Geometry: see drawing. Coordinates: mm, zero at the bounding-box minimum. A direction names the side the tool comes from. Coordinates: 2 decimals unless noted, no trailing zeros. Loops run counter-clockwise (first coordinate to the right, second up) from the corner with the lowest first, then second, coordinate; pieces in that order, holes last.
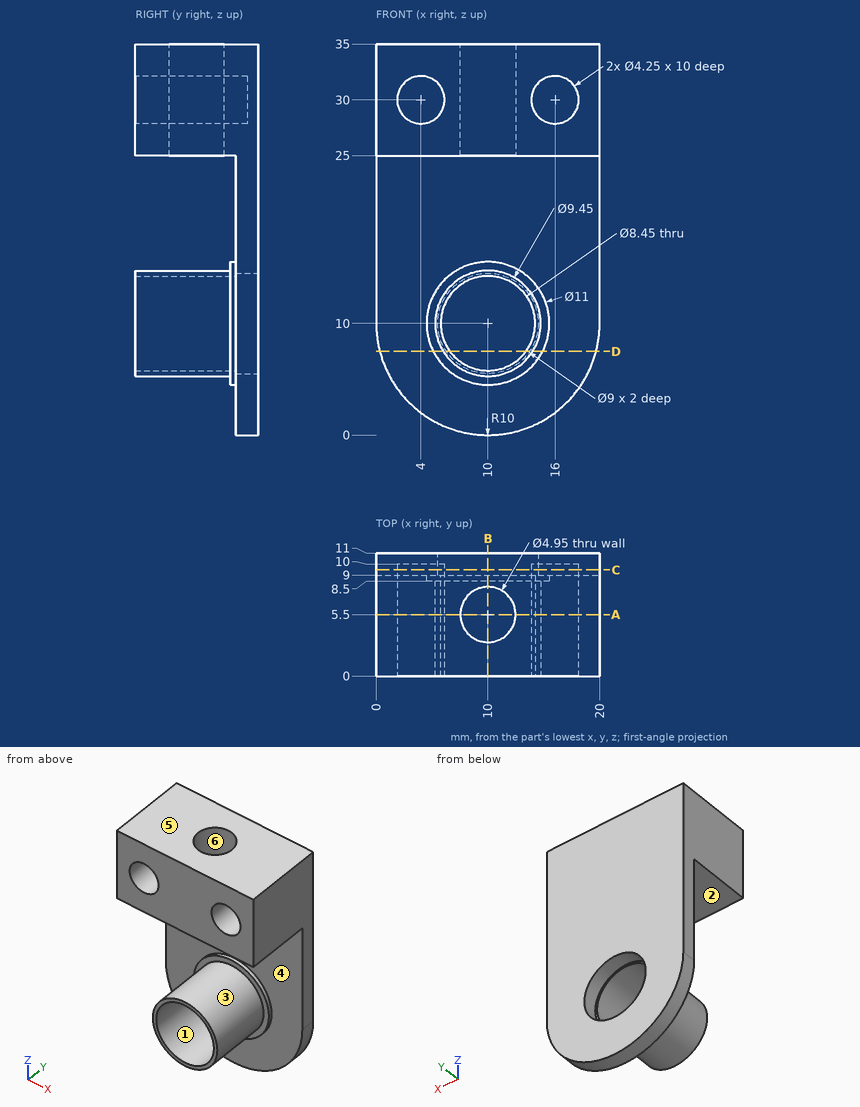
Item 1: Section query C-C (y = 9.5). Output: boundary loops of the cut face in (x, z) (3 decimals).
Result:
outline: (0, 10) arc R10 ccw to (20, 10) - (20, 35) - (0, 35) - close; hole circle Ø4.25 at (4, 30); hole circle Ø9 at (10, 10); hole circle Ø4.25 at (16, 30)
Item 2: Reachability of the marked faces 1, 2 and 3 from +Z, -Z, +X, -X, +Y, -Y: full face, straight path, thin tool, end or side. Return the list, or none.
Result:
face 1: +Y, -Y
face 2: +X, -X, -Y
face 3: -Y
Item 3: Mould query, pull axis Z, two halves, no side actions, for the marked faces 4, 5 and 6. Classes: +Z half, -Z half, draft (parallel to the pull), parting line (faces both ways), or undercut.
Result:
face 4: undercut
face 5: +Z half
face 6: draft
Item 4: Line query: L1, parallel to Z at x = 10, y = 9.95; L2, parallel to Z at x = 11.5, y = 8.75; L3, parallel to Z at x = 16, y = 8.25 (3 decimals). Output: solid intervals per line, ascending.
Result:
L1: z = 0 to 5.5, 14.5 to 35
L2: z = 4.71 to 6.05, 13.95 to 15.29, 25 to 35
L3: z = 25 to 27.875, 32.125 to 35
Item 5: Contact query for flat-ended pins moving along their axis: P1, Ø2, axis at x = 10, y = 2.5, coming from the -Z side (3 decimals); P2, Ø3.5, axis at x = 16, z = 29, coming from the -Y side; P3, Ø4.5, axis at x = 8, z = 9.5, coming from the +Y side; P4, Ø4, axis at x = 16, z = 30, coming from the -Y side. Output: stop coordinate, or through.
Result:
P1: stops at z = 5.275
P2: stops at y = 0
P3: stops at y = 9
P4: stops at y = 10
Item 6: Section query A-A (y = 5.5). Output: boundary loops of the cut face in (x, z) (3 decimals).
Result:
outline: (0, 25) - (7.525, 25) - (7.525, 35) - (0, 35) - close; circle Ø9.45 at (10, 10); (12.475, 25) - (20, 25) - (20, 35) - (12.475, 35) - close; hole circle Ø4.25 at (4, 30); hole circle Ø8.45 at (10, 10); hole circle Ø4.25 at (16, 30)
Item 7: Section query B-B (x = 10). Output: boundary loops of the cut face in (y, z) (3 decimals), then the cut area to 3 significant figures.
Result:
outline: (0, 5.275) - (8.5, 5.275) - (8.5, 4.5) - (9, 4.5) - (9, 0) - (11, 0) - (11, 5.5) - (9, 5.5) - (9, 5.775) - (0, 5.775) - close; (0, 14.225) - (9, 14.225) - (9, 14.5) - (11, 14.5) - (11, 35) - (7.975, 35) - (7.975, 25) - (9, 25) - (9, 15.5) - (8.5, 15.5) - (8.5, 14.725) - (0, 14.725) - close; (0, 25) - (3.025, 25) - (3.025, 35) - (0, 35) - close
area: 102 mm2
Item 8: Section query D-D (z = 7.5). Output: boundary loops of the cut face in (x, y), then the cut area to 3 significant figures.
Result:
outline: (0.32, 9) - (5.1, 9) - (5.1, 8.5) - (5.99, 8.5) - (5.99, 0) - (6.59, 0) - (6.59, 9) - (6.26, 9) - (6.26, 11) - (0.32, 11) - close; (13.41, 0) - (14.01, 0) - (14.01, 8.5) - (14.9, 8.5) - (14.9, 9) - (19.68, 9) - (19.68, 11) - (13.74, 11) - (13.74, 9) - (13.41, 9) - close
area: 35.5 mm2
